```python
from build123d import *

# Parameters (mm, degrees)
SKETCH_1_W      = 40
SKETCH_1_H      = 3
EXTRUDE_1_DEPTH = 22.5
SKETCH_2_R      = 10
EXTRUDE_2_DEPTH = 3


with BuildPart() as part:
    # 스케치1 → 보스-돌출1 (new, symmetric)
    with BuildSketch(Plane(origin=(0, 0, 0), x_dir=(0, 0, -1), z_dir=(1, 0, 0))):
        with Locations((0, 1.5)):
            Rectangle(SKETCH_1_W, SKETCH_1_H)
    extrude(amount=EXTRUDE_1_DEPTH, both=True)

    # 스케치2 → 보스-돌출2 (add)
    with BuildSketch(Plane(origin=(22.5, 0, 0), x_dir=(0, 0, -1), z_dir=(1, 0, 0))):
        with BuildLine():
            Line((-20, 31), (-20, 0))
            Line((-20, 0), (20, 0))
            Line((20, 0), (20, 31))
            ThreePointArc((20, 31), (0, 51), (-20, 31))
        make_face()
        with Locations((0, 31)):
            Circle(SKETCH_2_R, mode=Mode.SUBTRACT)
    extrude_2 = extrude(amount=EXTRUDE_2_DEPTH)

    # 대칭 복사1: 보스-돌출2 across plane
    add(extrude_2.mirror(Plane(origin=(0, 0, 0), x_dir=(0, 0, 1), z_dir=(1, 0, 0))))


solid = part.part
```
Work out the finished part from the listing and answer in its coordinate system (mm). A direction names the side the tool comes from. Give positions to 0.01 mm unless a question says otherwise; leave off trailing zeros. Order: outer loops, then holes, each group sorted by start corner. A loop starts at its lowest first (then second) coordinate and runs counter-clockwise, first axis right, second up. Notation, with made-up numbers: (4, 53.25) -> (19, 53.25) arc R10 ccw to (19, 71.25) -> close; hole circle Ø2 at (84, -21.5). An arc over 180 degrees is marked (long way). Answer as CSV lines item,"result". Start each with the question number.
(1) Section A-A, the plane z = 0 is taken. Write down the section's boundary in (x, y).
(2) Section B-B, the plane y = 18.5 is taken. Write down the section's boundary in (x, z).
(3) Which of the six approach directions +Z, -Z, +X, -X, +Y, -Y give full straight-line access (tool end or side, diameter ignored) to faces 1 (the flat face through (-22.5, 22, 5)), 2 (the flat face through (-25.5, 20, 0))?
(4) For a pull along X with two mould halves and no side action, classify faces 3 (the flat face through (25.5, 20, 0)), 4 (the cylindrical face through (24, 51, 0)), 5 (the flat face through (0, 3, 0)) as released by +X, released by -X, zero draft, split by the parting line, or undercut.
(5) Section D-D, the plane y = 25.5 is taken. Write down the section's boundary in (x, z).
(6) Section C-C, the plane z = -12 is taken. Write down the section's boundary in (x, y), plus the area to 3 significant figures.
(7) Consider line 1 along Y through (x, z) = (23.2, 0); line 2 along X through (y, z) = (10, 4); line 3 along Y through (x, z) = (-6, -6). Determine where each line is inside the solid, lowest interval first.
(8) Each of these flat-tipped pins is pushed along its axis until it touches: pin 1 Ø5 at (x, z) = (15, 14.5) entering from -Y; pin 2 Ø20 at (x, z) = (4, -3) entering from +Y. Where does it stop, or does it pass through?
Entries:
1,outline,"(-25.5, 0) -> (25.5, 0) -> (25.5, 21) -> (22.5, 21) -> (22.5, 3) -> (-22.5, 3) -> (-22.5, 21) -> (-25.5, 21) -> close; (-25.5, 41) -> (-22.5, 41) -> (-22.5, 51) -> (-25.5, 51) -> close; (22.5, 41) -> (25.5, 41) -> (25.5, 51) -> (22.5, 51) -> close"
2,outline,"(-25.5, -20) -> (-22.5, -20) -> (-22.5, 20) -> (-25.5, 20) -> close; (22.5, -20) -> (25.5, -20) -> (25.5, 20) -> (22.5, 20) -> close"
3,face 1,"+Z, -Z, +Y"
3,face 2,"+Z, -Z, -X, +Y, -Y"
4,face 3,"released by +X"
4,face 4,"zero draft"
4,face 5,"undercut"
5,outline,"(-25.5, -20) -> (-22.5, -20) -> (-22.5, -8.35) -> (-25.5, -8.35) -> close; (-25.5, 8.35) -> (-22.5, 8.35) -> (-22.5, 20) -> (-25.5, 20) -> close; (22.5, -20) -> (25.5, -20) -> (25.5, -8.35) -> (22.5, -8.35) -> close; (22.5, 8.35) -> (25.5, 8.35) -> (25.5, 20) -> (22.5, 20) -> close"
6,outline,"(-25.5, 0) -> (25.5, 0) -> (25.5, 47) -> (22.5, 47) -> (22.5, 3) -> (-22.5, 3) -> (-22.5, 47) -> (-25.5, 47) -> close"
6,area,"417 mm²"
7,line 1,"0 to 21, 41 to 51"
7,line 2,"-25.5 to -22.5, 22.5 to 25.5"
7,line 3,"0 to 3"
8,pin 1,"y = 0"
8,pin 2,"y = 3"
